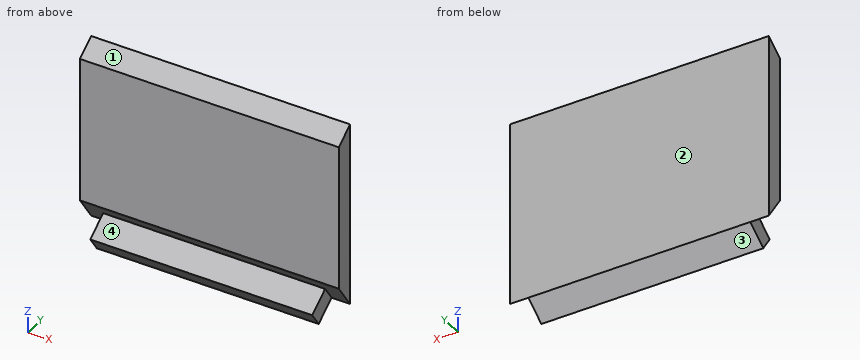
```python
from build123d import *

# Parameters (mm, degrees)
BOSS_EXTRUDE2_DEPTH = 44.45
SKETCH4_W           = 76.2
SKETCH4_H           = 6.35
BOSS_EXTRUDE3_DEPTH = 8.89


with BuildPart() as part:
    # Sketch2 → Boss-Extrude2 (new body, symmetric)
    with BuildSketch(Plane(origin=(0, 0, 0), x_dir=(0, 0, -1), z_dir=(1, 0, 0))):
        Polygon((22.681260157, -3.175), (31.75, 3.175), (-31.75, 3.175), (-27.303682132, -3.175), align=None)
    extrude(amount=BOSS_EXTRUDE2_DEPTH, both=True)

    # Sketch4 → Boss-Extrude3 (add)
    with BuildSketch(Plane(origin=(0, -12.787163377, -8.953668189), x_dir=(1, 0, 0), z_dir=(0, -0.819152044, -0.573576436))):
        with Locations((0, -24.654182592)):
            Rectangle(SKETCH4_W, SKETCH4_H)
    extrude(amount=BOSS_EXTRUDE3_DEPTH)


solid = part.part
```
The model under review builds one solid part; all positions refer to its coordinate system, in mm. Face numbers are marked on the shaded views. Coordinates: 2 decimals unless noted, no trailing zeros. Order: outer loops, then holes, each group sorted by start corner. A loop starts at its lowest first (then second) coordinate and runs counter-clockwise, first axis right, second up. Notation, with made-up numbers: M 13,-0.5 L 35,-0.5 A26 cw 35,28.5 Z; hole C 20,19.5 d5. An arc over 180 degrees is marked long. One line per question, with ' | ' between items.
(1) Add section B-B, the plane y = -1.5. Write out the cut boundary in (x, z).
Geometry results:
outline: M -44.45,-25.07 L 44.45,-25.07 L 44.45,28.48 L -44.45,28.48 Z; M -38.1,-35.02 L 38.1,-35.02 L 38.1,-27.27 L -38.1,-27.27 Z
(2) For probe 1 along Y at (x, z) = (-29.5, -20.5) (3 decimals); probe 2 along Z at (x, y) = (25.5, -2); probe 3 along Z at (x, y) = (26, -2.25), list the stretches that pass through material, from the lowest coordinate up. Write a range as from..to.
Geometry results:
probe 1: y = -3.175..3.175 | probe 2: z = -35.37..-27.62, -24.36..28.13 | probe 3: z = -35.55..-27.8, -24..27.95
(3) Insertion check: pin 1 (5 mm diameter, centred on x = -20.5, y = -6, fed in from -Z); pin 2 (1.5 mm diameter, centred on x = 1, y = 1.5, fed in from +Z); pin 3 (2 mm diameter, centred on x = 8.5, y = -1, fed in from +Z). Each pin has a flat end and moves straight along its axis. Give the tip position at first contact, or say it passes through.
Geometry results:
pin 1: stops at z = -36.85 | pin 2: stops at z = 31.1 | pin 3: stops at z = 29.53
(4) Add section C-C, the plane z = -18. Write out the cut boundary in (x, y) (3 decimals).
Geometry results:
outline: M -44.45,-3.175 L 44.45,-3.175 L 44.45,3.175 L -44.45,3.175 Z
(5) Add section A-A, the plane x = 10. Write out the cut boundary in (y, z) (3 decimals).
Geometry results:
outline: M -7.749,-31.647 L -4.107,-36.849 L 3.175,-31.75 L 3.175,31.75 L -3.175,27.304 L -3.175,-22.681 L -0.467,-26.548 Z
(6) The part is to be moulded in two halves that separate along Z. For the marked faces 1, 2, 3 and 4, say which applies: +Z half, -Z half, draft (parallel to the pull), parting line (faces both ways), or undercut.
Geometry results:
face 1: +Z half | face 2: draft | face 3: -Z half | face 4: undercut
